Verification items for the finished model (mm, model axes). Face numbers are marked on the shaded views. A direction names the side the tool comes from. Coordinates: 2 decimals unless noted, no trailing zeros. Loops run counter-clockwise (first coordinate to the right, second up) from the corner with the lowest first, then second, coordinate; pieces in that order, holes last. Notation, with made-up numbers: (52, 42.25) - (62, 42.25) arc R17 cw to (62, 63.25) - close; hole circle Ø5 at (72, 17). An arc over 180 degrees is marked (long way). One line per item, written item: value. Start each with the question number.
(1) Set-up check for the marked faces 4 and 5: record each of +Z, -Z, +X, -X, +Y, -Y from which the full face is reachable in a straight line by a thin tool's end or side.
(2) Draft check along X on the marked faces 1, 2 and 3. Enter one of: +X half, -X half, draft (parallel to the pull), parting line (faces both ways), or undercut.
(3) Section check B-B (y = -29). Record the boundary of the cut face in (x, z), plus the area to 3 significant figures.
(4) Gauge pin test, flat ends, axial feed: P1, Ø3, axis at x = 85, y = -28.5, coming from the -Z side; P2, Ø3, axis at x = 46.5, y = -35.5, coming from the +Z side. Record the tip position at first contact, or that the pin passes through.
(5) Thickness scan on probe 1 along X at (y, z) = (-43.5, 14.75); probe 2 along Y at (x, z) = (15, 13.75); probe 3 along Z at (x, y) = (14.5, -12). Record the ranges inside material, lowest first. Write a range as [from, to].
(6) Section check A-A (z = 10.75). Record the boundary of the cut face in (x, y), plus the area to 3 significant figures.
(7) Section check C-C (x = 32.5). Record the boundary of the cut face in (y, z), plus the area to 3 significant figures.
```python
from build123d import *

# Parameters (mm, degrees)
SKETCH1_W           = 170
SKETCH1_H           = 70
BOSS_EXTRUDE1_DEPTH = 20
SKETCH2_W           = 165.280045526
SKETCH2_H           = 65.058846286
CUT_EXTRUDE1_DEPTH  = 18
CHAMFER1_SIZE       = 3


with BuildPart() as part:
    # Sketch1 → Boss-Extrude1 (new body)
    with BuildSketch(Plane.XY):
        with Locations((85, -35)):
            Rectangle(SKETCH1_W, SKETCH1_H)
    extrude(amount=BOSS_EXTRUDE1_DEPTH)

    # Sketch2 → Cut-Extrude1 (cut)
    with BuildSketch(Plane.XY.offset(20)):
        with Locations((85.08493322, -35.169866439)):
            Rectangle(SKETCH2_W, SKETCH2_H)
    extrude(amount=-CUT_EXTRUDE1_DEPTH, mode=Mode.SUBTRACT)

    # Chamfer1
    chamfer1_edges = [part.edges().sort_by_distance(p)[0] for p in [
        (0, 0, 10),
        (170, 0, 10),
        (170, -70, 10),
        (0, -70, 10),
    ]]
    chamfer(chamfer1_edges, length=CHAMFER1_SIZE)


solid = part.part
```
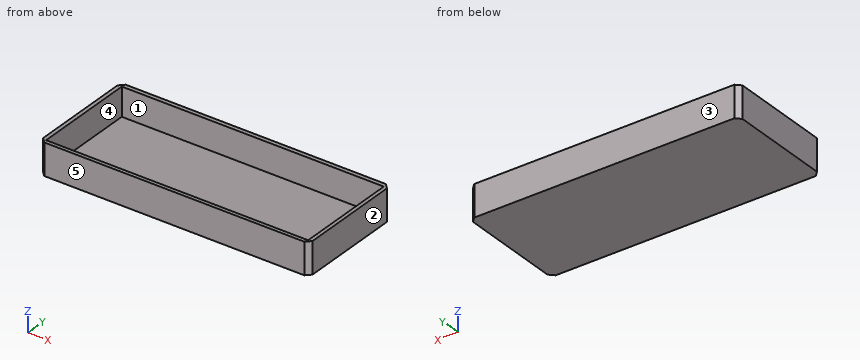
Responses:
1. face 4: +Z
1. face 5: +Z, -Z, +X, -X, -Y
2. face 1: undercut
2. face 2: +X half
2. face 3: draft
3. outline: (0, 0) - (170, 0) - (170, 20) - (167.72, 20) - (167.72, 2) - (2.44, 2) - (2.44, 20) - (0, 20) - close
3. area: 425 mm²
4. P1: stops at z = 0
4. P2: stops at z = 2
5. probe 1: x = [0, 2.44], [167.72, 170]
5. probe 2: y = [-70, -67.7], [-2.64, 0]
5. probe 3: z = [0, 2]
6. outline: (0, -67) - (3, -70) - (167, -70) - (170, -67) - (170, -3) - (167, 0) - (3, 0) - (0, -3) - close; hole (2.44, -67.7) - (167.72, -67.7) - (167.72, -2.64) - (2.44, -2.64) - close
6. area: 1,130 mm²
7. outline: (-70, 0) - (0, 0) - (0, 20) - (-2.64, 20) - (-2.64, 2) - (-67.7, 2) - (-67.7, 20) - (-70, 20) - close
7. area: 229 mm²
